Read the model definition and answer for the solid it produces. Units are mm, in the model's axes. Face numbers are marked on the shaded views. A direction names the side the tool comes from. Coordinates: 2 decimals unless noted, no trailing zeros. Write each loop counter-clockwise with the first axis right and the second up, starting at its lowest first coordinate (ties: lowest second). Pieces come first, ordered by that corner, then holes. Notation, with made-up numbers: M -3.5,4 L 12.5,4 A19 ccw 12.5,8 Z; hole C -26,84.25 d4. An arc over 180 degrees is marked long. Use a Markdown table: item, result. Add a question column.
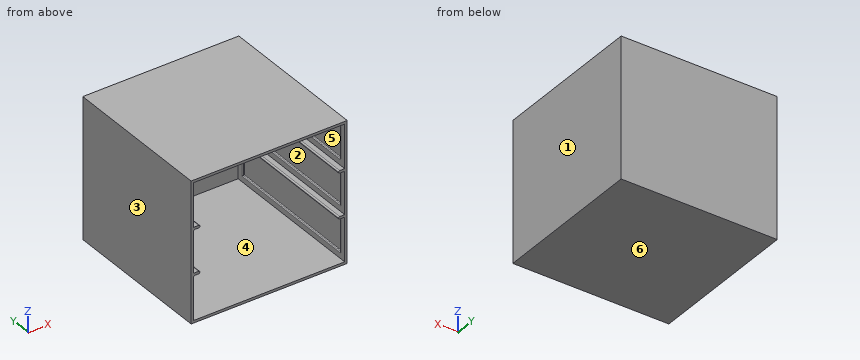
from build123d import *

# Parameters (mm, degrees)
F0_W      = 125
F0_H      = 122
F1_DEPTH  = 2
F2_W      = 121
F2_H      = 2
F2_W_2    = 2
F2_H_2    = 120
F3_DEPTH  = 108
F4_W      = 125
F4_H      = 122
F5_DEPTH  = 2
F6_W      = 4.9999992847
F6_H      = 1
F6_W_2    = 5
F7_DEPTH  = 120
F8_DEPTH  = 1
F9_W      = 111
F9_H      = 25
F9_W_2    = 111.000007391
F9_H_2    = 24.000007391
F9_W_3    = 111.0000030398
F9_H_3    = 25.0000030398
F11_DEPTH = 1.2
F10_W     = 111
F10_H     = 25
F10_H_2   = 24
F12_DEPTH = 1.2
F13_R     = 0.99999
F14_R     = 0.59999


# Not quite as in the source:
# - a fillet or chamfer is up to 0.001 mm smaller than in the source, because OpenCascade refuses the exact size
# - a feature names something its author has since deleted; it is built from what else it names


with BuildPart() as f1:
    # F0 (on Top) → F1 (new body)
    with BuildSketch(Plane.XY):
        Rectangle(F0_W, F0_H)
    extrude(amount=F1_DEPTH)

    # F2 (on face) → F3 (join)
    with BuildSketch(Plane.XY.offset(2)):
        with Locations((0, 60)):
            Rectangle(F2_W, F2_H)
        with Locations((-61.5, 60)):
            Rectangle(F2_W_2, F2_H)
        with Locations((-61.5, -1)):
            Rectangle(F2_W_2, F2_H_2)
        with Locations((61.5, -1)):
            Rectangle(F2_W_2, F2_H_2)
        with Locations((61.5, 60)):
            Rectangle(F2_W_2, F2_H)
    extrude(amount=F3_DEPTH)

    # F4 (on face) → F5 (join)
    with BuildSketch(Plane.XY.offset(110)):
        Rectangle(F4_W, F4_H)
    extrude(amount=F5_DEPTH)

    # F6 (on face) → F7 (join)
    with BuildSketch(Plane.XZ.offset(61)):
        with Locations((-58.0000003576, 74.5)):
            Rectangle(F6_W, F6_H)
        with Locations((-58.0000003576, 73.5)):
            Rectangle(F6_W, F6_H)
        with Locations((-58.0000003576, 38.5)):
            Rectangle(F6_W, F6_H)
        with Locations((-58.0000003576, 37.5)):
            Rectangle(F6_W, F6_H)
        with Locations((58, 74.5)):
            Rectangle(F6_W_2, F6_H)
        with Locations((58, 73.5)):
            Rectangle(F6_W_2, F6_H)
        with Locations((58, 38.5)):
            Rectangle(F6_W_2, F6_H)
        with Locations((58, 37.5)):
            Rectangle(F6_W_2, F6_H)
    extrude(amount=-F7_DEPTH)

    # F8 (add): a face of the model
    f8_faces = [f1.faces().sort_by_distance(p)[0] for p in [
        (-60.821637703, -61, 56),
    ]]
    extrude(f8_faces, amount=F8_DEPTH)

    # F9 (on face) → F11 (cut)
    with BuildSketch(Plane.YZ.offset(-60.5)):
        with Locations((-1.5, 92.5)):
            Rectangle(F9_W, F9_H)
        with Locations((-1.5, 56)):
            Rectangle(F9_W_2, F9_H_2)
        with Locations((-1.5, 19.5)):
            Rectangle(F9_W_3, F9_H_3)
    extrude(amount=-F11_DEPTH, mode=Mode.SUBTRACT)

    # F10 (on face) → F12 (cut)
    with BuildSketch(Plane(origin=(60.5, 0, 0), x_dir=(0, -1, 0), z_dir=(-1, 0, 0))):
        with Locations((1.5, 92.5)):
            Rectangle(F10_W, F10_H)
        with Locations((1.5, 56)):
            Rectangle(F10_W, F10_H_2)
        with Locations((1.5, 19.5)):
            Rectangle(F10_W, F10_H)
    extrude(amount=-F12_DEPTH, mode=Mode.SUBTRACT)

    # F13 (radius 1 in the source; OpenCascade refuses exactly that, so slightly less here)
    f13_edges = [f1.edges().sort_by_distance(p)[0] for p in [
        (55.5, -1.5, 75),
        (55.5, -1.5, 73),
        (55.5, -1.5, 39),
        (55.5, -1.5, 37),
        (-55.500001, -1.5, 75),
        (-55.500001, -1.5, 73),
        (-55.500001, -1.5, 39),
        (-55.500001, -1.5, 37),
        (-60.5, -1.5, 73),
        (-60.5, -1.5, 37),
        (60.5, -1.5, 73),
        (60.5, -1.5, 37),
    ]]
    fillet(f13_edges, radius=F13_R)

    # F14 (radius 0.6 in the source; OpenCascade refuses exactly that, so slightly less here)
    f14_edges = [f1.edges().sort_by_distance(p)[0] for p in [
        (-61.7, 54, 92.5),
        (-61.7, -1.5, 105),
        (-61.7, -57, 92.5),
        (-61.7, -1.5, 80),
        (-60.5, -1.5, 80),
        (-60.5, -57, 92.5),
        (-60.5, -1.5, 105),
        (-60.5, 54, 92.5),
        (-61.7, 54.000004, 56),
        (-61.7, -1.5, 68.000004),
        (-61.7, -57.000004, 56),
        (-61.7, -1.5, 43.999996),
        (-60.5, -1.5, 68.000004),
        (-60.5, -57.000004, 56),
        (-60.5, 54.000004, 56),
        (-60.5, -1.5, 43.999996),
        (-61.7, -1.5, 6.999998),
        (-61.7, 54.000002, 19.5),
        (-61.7, -1.5, 32.000002),
        (-61.7, -57.000002, 19.5),
        (-60.5, -1.5, 32.000002),
        (-60.5, -57.000002, 19.5),
        (-60.5, -1.5, 6.999998),
        (61.7, -57, 19.5),
        (61.7, -1.5, 32),
        (61.7, 54, 19.5),
        (61.7, -1.5, 7),
        (61.7, -1.5, 68),
        (61.7, 54, 56),
        (61.7, -1.5, 44),
        (61.7, -57, 56),
        (61.7, -1.5, 105),
        (61.7, 54, 92.5),
        (61.7, -1.5, 80),
        (61.7, -57, 92.5),
        (60.5, -1.5, 105),
        (60.5, 54, 92.5),
        (60.5, -57, 92.5),
        (61.1, 54, 80),
        (61.1, -57, 80),
        (60.5, -1.5, 80),
        (60.5, -1.5, 68),
        (60.5, -57, 56),
        (60.5, 54, 56),
        (60.5, -1.5, 44),
        (60.5, 54, 19.5),
        (60.5, -1.5, 32),
        (60.5, -1.5, 7),
        (60.5, -57, 19.5),
    ]]
    fillet(f14_edges, radius=F14_R)


solid = f1.part
Item 1: This flat-tipped pin is pushed along its axis until it touches: pin 1 (1.5 mm diameter, centred on x = -15, z = 84, fed in from -Y). Where does it stop, or does it pass through?
Item 2: Consider probe 1 along X at (y, z) = (3, 56); probe 2 along Z at (x, y) = (-29, 24.5); probe 3 along X at (y, z) = (-29.5, 70.5). Determine where each line is inside the solid, lowest interval first.
Item 3: For the marked faces 5 and 6, determine the directions among +Z, -Z, +X, -X, +Y, -Y from which every point of the face is accessible in a straight line to the end or side of a thin tool.
Item 4: Find section C-C on z = 77. Give the vertices of the cut face in (x, y), then the cut area to 3 significant figures.
Item 5: Find section A-A on x = 35. Give the vertices of the cut face in (y, z), then the cut area to 3 significant figures.
Item 6: Determine the mould class of the marked faces 1, 2, 3 and 4 for opening direction X: pulls with the +X half, pulls with the -X half, needs draft (parallel to the pull), parting line crosses it, or undercut.
Geometry says:
| question | item | result |
|---|---|---|
| 1 | pin 1 | stops at y = 59 |
| 2 | probe 1 | x = -62.5 to -61.7, 61.7 to 62.5 |
| 2 | probe 2 | z = 0 to 2, 110 to 112 |
| 2 | probe 3 | x = -62.5 to -60.5, 60.5 to 62.5 |
| 3 | face 5 | none |
| 3 | face 6 | -Z, +X, -X, +Y, -Y |
| 4 | outline | M -62.5,-62 L -60.5,-62 L -60.5,59 L 60.5,59 L 60.5,-62 L 62.5,-62 L 62.5,61 L -62.5,61 Z |
| 4 | area | 734 mm2 |
| 5 | outline | M -62,0 L 61,0 L 61,112 L -62,112 L -62,110 L 59,110 L 59,2 L -62,2 Z |
| 5 | area | 708 mm2 |
| 6 | face 1 | pulls with the +X half |
| 6 | face 2 | undercut |
| 6 | face 3 | pulls with the -X half |
| 6 | face 4 | undercut |
